The figure shows three views and two pictorial views of one solid part (mm, origin at its lowest corner). Answer the questions. Coordinates: 2 decimals unless noted, no trailing zeros. Order: outer loops, then holes, each group sorted by start corner. A loop starts at its lowest first (then second) coordinate and runs counter-clockwise, first axis right, second up. Notation, with made-up numbers: M -32.75,16.25 L -3.75,16.25 A25 ccw -3.75,51.25 Z; hole C -23,40.25 d8. An arc over 180 degrees is marked long. Use a Markdown table: item, result.
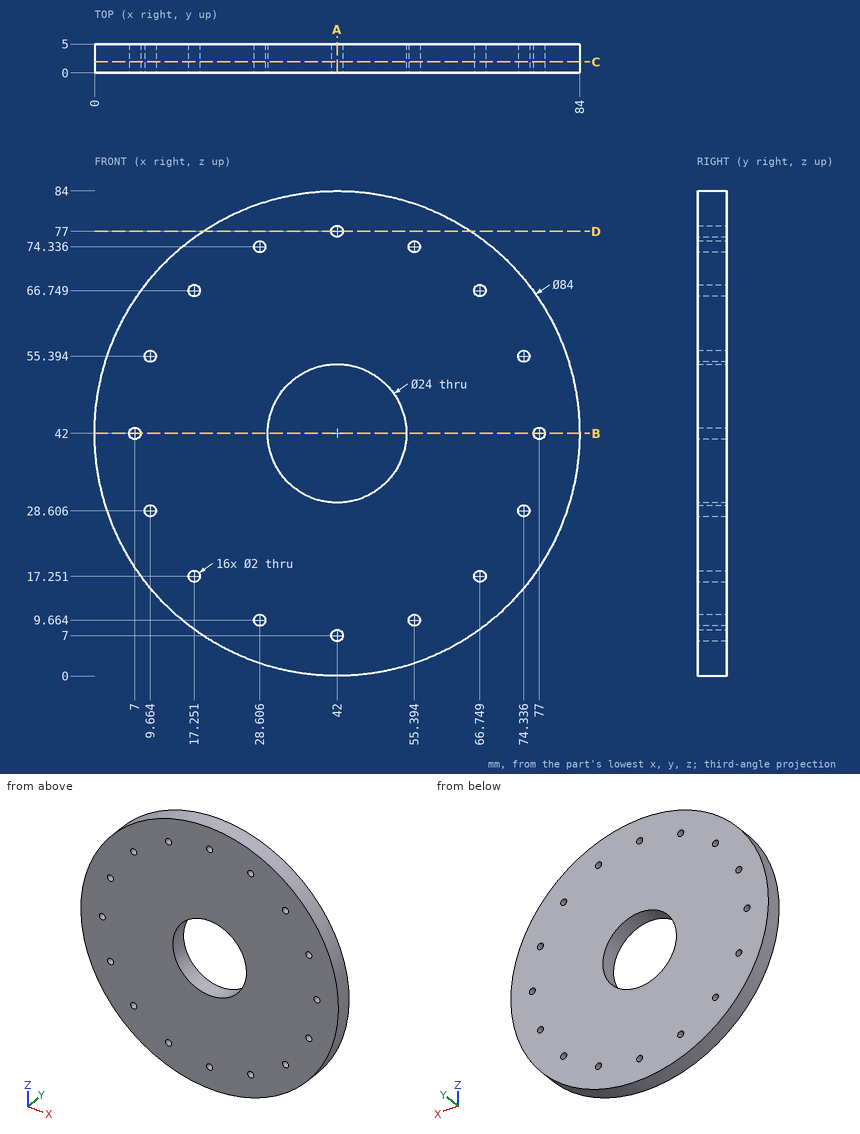
1. Section A-A on x = 42 is taken. Determine the outline of the cut face in (y, z).
Answers below:
| item | result |
|---|---|
| outline | M 0,0 L 5,0 L 5,6 L 0,6 Z; M 0,8 L 5,8 L 5,30 L 0,30 Z; M 0,54 L 5,54 L 5,76 L 0,76 Z; M 0,78 L 5,78 L 5,84 L 0,84 Z |
2. Find the intervals of material crossed by probe 1 along X at (y, z) = (3, 42); probe 2 along Z at (x, y) = (73.5, 4.3) (1 decimal); probe 3 along X at (y, z) = (1.2, 41.5) (1 decimal), in increasing order.
Answers below:
| item | result |
|---|---|
| probe 1 | 0 to 6, 8 to 30, 54 to 76, 78 to 84 |
| probe 2 | 14.2 to 28.1, 29.2 to 54.8, 55.9 to 69.8 |
| probe 3 | 0 to 6.1, 7.9 to 30, 54 to 76.1, 77.9 to 84 |
3. Section B-B on z = 42 is taken. Determine the outline of the cut face in (x, y).
Answers below:
| item | result |
|---|---|
| outline | M 0,0 L 6,0 L 6,5 L 0,5 Z; M 8,0 L 30,0 L 30,5 L 8,5 Z; M 54,0 L 76,0 L 76,5 L 54,5 Z; M 78,0 L 84,0 L 84,5 L 78,5 Z |
4. Section D-D on z = 77 is taken. Determine the outline of the cut face in (x, y), then the cut area to 3 significant figures.
Answers below:
| item | result |
|---|---|
| outline | M 18.78,0 L 41,0 L 41,5 L 18.78,5 Z; M 43,0 L 65.22,0 L 65.22,5 L 43,5 Z |
| area | 222 mm² |
5. Flat-ended cylindrical pins translate along their axes: P1, Ø3, axis at y = 2.5, z = 9, coming from the -X side; P2, Ø1.5, axis at y = 2.5, z = 9, coming from the -X side (1 decimal); P3, Ø3, axis at x = 64.5, y = 2, coming from the -Z side. Find the tip coordinate at first contact, or state that the pin passes through.
Answers below:
| item | result |
|---|---|
| P1 | x = 14.22 |
| P2 | x = 15.1 |
| P3 | z = 5.63 |
6. Section C-C on y = 1.9 is taken. Give the number of separate pieces and of enclosed holes in the cut face, then the cut area to 3 significant figures.
Answers below:
| item | result |
|---|---|
| separate pieces | 1 |
| enclosed holes | 17 |
| area | 5,040 mm² |
